Check sheet for the modelled part. Datum: model origin and axes. Units: mm. A direction names the side the tool comes from. Round coordinates to 2 decimals unless told otherwise and drop trailing zeros. Loops run counter-clockwise (first coordinate to the right, second up) from the corner with the lowest first, then second, coordinate; pieces in that order, holes last. Notation, with made-up numbers: (68.25, 72.5) -> (86.25, 72.5) arc R23 ccw to (86.25, 84.5) -> close; hole circle Ø5 at (42.25, -20). An arc over 180 degrees is marked (long way). Use one line per item in the form item = value. Start each with the question number.
(1) Draft check along Y on faces 1 (the flat face through (40.417, -66, 7)), 2 (the flat face through (42.917, -33, 8)), 3 (the flat face through (47, -54.781, 8)). Enter one of: released by +Y, released by -Y, zero draft, split by the parting line, or undercut.
(2) Go/stop test with flat-tipped pins: pin 1 (10 mm diameter, centred on x = 53.92, y = -49.38, fed in from +Z); pin 2 (4.5 mm diameter, centred on y = -59.5, z = 5.5, fed in from -X); pin 3 (5.5 mm diameter, centred on y = -29, z = 5, fed in from +X); pin 4 (3.5 mm diameter, centred on y = -35, z = 7, fed in from -X). Record where each tip stops, or that it passes through.
(3) Material ranges on probe 1 along X at (y, z) = (-62.5, 6); probe 2 along X at (y, z) = (-61, 10); probe 3 along X at (y, z) = (-59.5, 7.5), recorded low to high. Write a range as [from, to].
(4) Sectioned sample at C-C (y = -37). Record the cut outline in (x, z), and give its area (4 significant figures).
(5) Set-up check for faces 4 (the flat face through (48, -62.281, 5.7)), 5 (the flat face through (12, -23, 3.75)), 6 (the flat face through (39, -45.781, 7)), 7 (the flat face through (55, -45.781, 7)), 8 (the flat face through (12, -23, 11.25)): record each of +Z, -Z, +X, -X, +Y, -Y from which the full face is reachable in a straight line by a thin tool's end or side.
(6) Sectioned sample at B-B (x = 8). Record the cut outline in (y, z), and give its area (4 significant figures).
(7) Sectioned sample at A-A (z = 7.5). Record the cut outline in (x, y) (3 decimals), and give its area (3 significant figures).
from build123d import *

# Parameters (mm, degrees)
SKETCH1_R           = 3.175
PUSHER_BASE_DEPTH   = 15
SKETCH3_R           = 1.95
SCREW_HOLE_DEPTH    = 7.5
SKETCH6_W           = 7.5
SKETCH6_H           = 26.5
PUSHER_HEAD_DEPTH   = 3.75
FILLET1_R           = 6
FILLET5_R           = 6
FILLET6_R           = 6
SKETCH8_W           = 92.5
SKETCH8_H           = 4.5
BOSS_EXTRUDE1_DEPTH = 7.5


with BuildPart() as part:
    # Sketch1 → pusher base (new body)
    with BuildSketch(Plane.XY):
        Polygon((59.166899441, -45.781018283), (51.666899441, -45.781018283), (41.666899441, -45.781018283), (34.166899441, -45.781018283), (34.166899441, -69.281018283), (40.416899441, -69.281018283), (40.416899441, -62.281018283), (52.916899441, -62.281018283), (52.916899441, -69.281018283), (59.166899441, -69.281018283), align=None)
        with Locations((39.416899441, -49.381018283)):
            Circle(SKETCH1_R, mode=Mode.SUBTRACT)
        with Locations((53.916899441, -49.381018283)):
            Circle(SKETCH1_R, mode=Mode.SUBTRACT)
    extrude(amount=PUSHER_BASE_DEPTH)

    # Sketch3 → screw hole (cut)
    with BuildSketch(Plane.XZ.offset(62.281018283)):
        with Locations(Location((46.666899441, 7.5, 0), (0, 0, 270))):
            Circle(SKETCH3_R)
    extrude(amount=-SCREW_HOLE_DEPTH, mode=Mode.SUBTRACT)

    # Sketch6 → pusher head (add, symmetric)
    with BuildSketch(Plane.XY.offset(7.5)):
        with Locations((46.666899441, -32.531018283)):
            Rectangle(SKETCH6_W, SKETCH6_H)
    extrude(amount=PUSHER_HEAD_DEPTH, both=True)

    # Fillet1
    # the kernel refuses this fillet: 6 mm, written as the material it takes off along each edge
    with BuildSketch(Plane(origin=(74.166899441, -45.781018283, 0), x_dir=(0, 0, 1), z_dir=(-1, 0, 0))) as fillet1_piece_1_section:
        with BuildLine():
            CenterArc((FILLET1_R, -FILLET1_R), FILLET1_R, 90, 90)
            Line((0, -FILLET1_R), (0, 0))
            Line((0, 0), (FILLET1_R, 0))
        make_face()
    fillet1_piece_1 = extrude(amount=55, mode=Mode.PRIVATE)
    fillet1_piece_1 = split(fillet1_piece_1, bisect_by=Plane(origin=(62.291899441, -45.824840722, 3.75), z_dir=(0, 0, 1)), keep=Keep.TOP, mode=Mode.PRIVATE)
    fillet1_piece_1 = split(fillet1_piece_1, bisect_by=Plane(origin=(50.416899441, -45.824840722, 4.566140917), z_dir=(1, 0, 0)), keep=Keep.TOP, mode=Mode.PRIVATE)
    add(fillet1_piece_1, mode=Mode.SUBTRACT)
    with BuildSketch(Plane(origin=(74.166899441, -45.781018283, 0), x_dir=(0, 0, 1), z_dir=(-1, 0, 0))) as fillet1_piece_2_section:
        with BuildLine():
            CenterArc((FILLET1_R, -FILLET1_R), FILLET1_R, 90, 90)
            Line((0, -FILLET1_R), (0, 0))
            Line((0, 0), (FILLET1_R, 0))
        make_face()
    fillet1_piece_2 = extrude(amount=55, mode=Mode.PRIVATE)
    fillet1_piece_2 = split(fillet1_piece_2, bisect_by=Plane(origin=(62.291899441, -47.230240291, 3.75), z_dir=(0, 0, -1)), keep=Keep.TOP, mode=Mode.PRIVATE)
    fillet1_piece_2 = split(fillet1_piece_2, bisect_by=Plane(origin=(50.416899441, -47.230240291, 1.136674626), z_dir=(1, 0, 0)), keep=Keep.TOP, mode=Mode.PRIVATE)
    add(fillet1_piece_2, mode=Mode.SUBTRACT)
    with BuildSketch(Plane(origin=(74.166899441, -45.781018283, 0), x_dir=(0, 0, 1), z_dir=(-1, 0, 0))) as fillet1_piece_3_section:
        with BuildLine():
            CenterArc((FILLET1_R, -FILLET1_R), FILLET1_R, 90, 90)
            Line((0, -FILLET1_R), (0, 0))
            Line((0, 0), (FILLET1_R, 0))
        make_face()
    fillet1_piece_3 = extrude(amount=55, mode=Mode.PRIVATE)
    fillet1_piece_3 = split(fillet1_piece_3, bisect_by=Plane(origin=(46.666899441, -47.230240291, 3.75), z_dir=(0, 0, -1)), keep=Keep.TOP, mode=Mode.PRIVATE)
    fillet1_piece_3 = split(fillet1_piece_3, bisect_by=Plane(origin=(50.416899441, -47.230240291, 1.136674626), z_dir=(-1, 0, 0)), keep=Keep.TOP, mode=Mode.PRIVATE)
    fillet1_piece_3 = split(fillet1_piece_3, bisect_by=Plane(origin=(42.916899441, -47.230240291, 1.136674626), z_dir=(1, 0, 0)), keep=Keep.TOP, mode=Mode.PRIVATE)
    add(fillet1_piece_3, mode=Mode.SUBTRACT)
    with BuildSketch(Plane(origin=(74.166899441, -45.781018283, 0), x_dir=(0, 0, 1), z_dir=(-1, 0, 0))) as fillet1_piece_4_section:
        with BuildLine():
            CenterArc((FILLET1_R, -FILLET1_R), FILLET1_R, 90, 90)
            Line((0, -FILLET1_R), (0, 0))
            Line((0, 0), (FILLET1_R, 0))
        make_face()
    fillet1_piece_4 = extrude(amount=55, mode=Mode.PRIVATE)
    fillet1_piece_4 = split(fillet1_piece_4, bisect_by=Plane(origin=(31.041899441, -45.824840722, 3.75), z_dir=(0, 0, 1)), keep=Keep.TOP, mode=Mode.PRIVATE)
    fillet1_piece_4 = split(fillet1_piece_4, bisect_by=Plane(origin=(42.916899441, -45.824840722, 4.566140917), z_dir=(-1, 0, 0)), keep=Keep.TOP, mode=Mode.PRIVATE)
    add(fillet1_piece_4, mode=Mode.SUBTRACT)
    with BuildSketch(Plane(origin=(74.166899441, -45.781018283, 0), x_dir=(0, 0, 1), z_dir=(-1, 0, 0))) as fillet1_piece_5_section:
        with BuildLine():
            CenterArc((FILLET1_R, -FILLET1_R), FILLET1_R, 90, 90)
            Line((0, -FILLET1_R), (0, 0))
            Line((0, 0), (FILLET1_R, 0))
        make_face()
    fillet1_piece_5 = extrude(amount=55, mode=Mode.PRIVATE)
    fillet1_piece_5 = split(fillet1_piece_5, bisect_by=Plane(origin=(31.041899441, -47.230240291, 3.75), z_dir=(0, 0, -1)), keep=Keep.TOP, mode=Mode.PRIVATE)
    fillet1_piece_5 = split(fillet1_piece_5, bisect_by=Plane(origin=(42.916899441, -47.230240291, 1.136674626), z_dir=(-1, 0, 0)), keep=Keep.TOP, mode=Mode.PRIVATE)
    add(fillet1_piece_5, mode=Mode.SUBTRACT)
    with BuildSketch(Plane(origin=(19.166899441, -45.781018283, 15), x_dir=(0, 0, -1), z_dir=(1, 0, 0))) as fillet1_piece_6_section:
        with BuildLine():
            CenterArc((FILLET1_R, -FILLET1_R), FILLET1_R, 90, 90)
            Line((0, -FILLET1_R), (0, 0))
            Line((0, 0), (FILLET1_R, 0))
        make_face()
    fillet1_piece_6 = extrude(amount=55, mode=Mode.PRIVATE)
    fillet1_piece_6 = split(fillet1_piece_6, bisect_by=Plane(origin=(31.041899441, -45.824840722, 11.25), z_dir=(0, 0, -1)), keep=Keep.TOP, mode=Mode.PRIVATE)
    fillet1_piece_6 = split(fillet1_piece_6, bisect_by=Plane(origin=(42.916899441, -45.824840722, 10.433859083), z_dir=(-1, 0, 0)), keep=Keep.TOP, mode=Mode.PRIVATE)
    add(fillet1_piece_6, mode=Mode.SUBTRACT)
    with BuildSketch(Plane(origin=(19.166899441, -45.781018283, 15), x_dir=(0, 0, -1), z_dir=(1, 0, 0))) as fillet1_piece_7_section:
        with BuildLine():
            CenterArc((FILLET1_R, -FILLET1_R), FILLET1_R, 90, 90)
            Line((0, -FILLET1_R), (0, 0))
            Line((0, 0), (FILLET1_R, 0))
        make_face()
    fillet1_piece_7 = extrude(amount=55, mode=Mode.PRIVATE)
    fillet1_piece_7 = split(fillet1_piece_7, bisect_by=Plane(origin=(31.041899441, -47.230240291, 11.25), z_dir=(0, 0, 1)), keep=Keep.TOP, mode=Mode.PRIVATE)
    fillet1_piece_7 = split(fillet1_piece_7, bisect_by=Plane(origin=(42.916899441, -47.230240291, 13.863325374), z_dir=(-1, 0, 0)), keep=Keep.TOP, mode=Mode.PRIVATE)
    add(fillet1_piece_7, mode=Mode.SUBTRACT)
    with BuildSketch(Plane(origin=(19.166899441, -45.781018283, 15), x_dir=(0, 0, -1), z_dir=(1, 0, 0))) as fillet1_piece_8_section:
        with BuildLine():
            CenterArc((FILLET1_R, -FILLET1_R), FILLET1_R, 90, 90)
            Line((0, -FILLET1_R), (0, 0))
            Line((0, 0), (FILLET1_R, 0))
        make_face()
    fillet1_piece_8 = extrude(amount=55, mode=Mode.PRIVATE)
    fillet1_piece_8 = split(fillet1_piece_8, bisect_by=Plane(origin=(50.416899441, -47.230240291, 13.863325374), z_dir=(-1, 0, 0)), keep=Keep.TOP, mode=Mode.PRIVATE)
    fillet1_piece_8 = split(fillet1_piece_8, bisect_by=Plane(origin=(46.666899441, -47.230240291, 11.25), z_dir=(0, 0, 1)), keep=Keep.TOP, mode=Mode.PRIVATE)
    fillet1_piece_8 = split(fillet1_piece_8, bisect_by=Plane(origin=(42.916899441, -47.230240291, 13.863325374), z_dir=(1, 0, 0)), keep=Keep.TOP, mode=Mode.PRIVATE)
    add(fillet1_piece_8, mode=Mode.SUBTRACT)
    with BuildSketch(Plane(origin=(19.166899441, -45.781018283, 15), x_dir=(0, 0, -1), z_dir=(1, 0, 0))) as fillet1_piece_9_section:
        with BuildLine():
            CenterArc((FILLET1_R, -FILLET1_R), FILLET1_R, 90, 90)
            Line((0, -FILLET1_R), (0, 0))
            Line((0, 0), (FILLET1_R, 0))
        make_face()
    fillet1_piece_9 = extrude(amount=55, mode=Mode.PRIVATE)
    fillet1_piece_9 = split(fillet1_piece_9, bisect_by=Plane(origin=(50.416899441, -45.824840722, 10.433859083), z_dir=(1, 0, 0)), keep=Keep.TOP, mode=Mode.PRIVATE)
    fillet1_piece_9 = split(fillet1_piece_9, bisect_by=Plane(origin=(62.291899441, -45.824840722, 11.25), z_dir=(0, 0, -1)), keep=Keep.TOP, mode=Mode.PRIVATE)
    add(fillet1_piece_9, mode=Mode.SUBTRACT)
    with BuildSketch(Plane(origin=(19.166899441, -45.781018283, 15), x_dir=(0, 0, -1), z_dir=(1, 0, 0))) as fillet1_piece_10_section:
        with BuildLine():
            CenterArc((FILLET1_R, -FILLET1_R), FILLET1_R, 90, 90)
            Line((0, -FILLET1_R), (0, 0))
            Line((0, 0), (FILLET1_R, 0))
        make_face()
    fillet1_piece_10 = extrude(amount=55, mode=Mode.PRIVATE)
    fillet1_piece_10 = split(fillet1_piece_10, bisect_by=Plane(origin=(50.416899441, -47.230240291, 13.863325374), z_dir=(1, 0, 0)), keep=Keep.TOP, mode=Mode.PRIVATE)
    fillet1_piece_10 = split(fillet1_piece_10, bisect_by=Plane(origin=(62.291899441, -47.230240291, 11.25), z_dir=(0, 0, 1)), keep=Keep.TOP, mode=Mode.PRIVATE)
    add(fillet1_piece_10, mode=Mode.SUBTRACT)

    # Fillet5
    fillet5_edges = [part.edges().sort_by_distance(p)[0] for p in [
        (46.666899441, -46.218869418, 11.25),
    ]]
    fillet(fillet5_edges, radius=FILLET5_R)

    # Fillet6
    fillet6_edges = [part.edges().sort_by_distance(p)[0] for p in [
        (46.666899441, -46.218869418, 3.75),
    ]]
    fillet(fillet6_edges, radius=FILLET6_R)

    # Sketch8 → Boss-Extrude1 (add)
    with BuildSketch(Plane(origin=(0, 0, 3.75), x_dir=(-1, 0, 0), z_dir=(0, 0, -1))):
        with Locations((3.333100559, -21.531018283)):
            Rectangle(SKETCH8_W, SKETCH8_H)
    extrude(amount=-BOSS_EXTRUDE1_DEPTH)


solid = part.part
Checks:
q1.face_1 = zero draft
q1.face_2 = undercut
q1.face_3 = released by -Y
q2.pin_1 = 15
q2.pin_2 = 34.17
q2.pin_3 = 50.42
q2.pin_4 = 42.92
q3.probe_1 = [34.17, 40.42], [52.92, 59.17]
q3.probe_2 = [34.17, 59.17]
q3.probe_3 = [34.17, 44.72], [48.62, 59.17]
q4.outline = (42.92, 3.75) -> (50.42, 3.75) -> (50.42, 11.25) -> (42.92, 11.25) -> close
q4.area = 56.25 mm2
q5.face_4 = +Z, -Z, -Y
q5.face_5 = -Z, +X, -X, +Y
q5.face_6 = +Z, -Z, -X
q5.face_7 = +Z, -Z, +X, +Y
q5.face_8 = +Z, +X, -X, +Y
q6.outline = (-23.78, 3.75) -> (-19.28, 3.75) -> (-19.28, 11.25) -> (-23.78, 11.25) -> close
q6.area = 33.75 mm2
q7.outline = (-49.583, -23.781) -> (42.917, -23.781) -> (42.917, -45.781) -> (34.167, -45.781) -> (34.167, -69.281) -> (40.417, -69.281) -> (40.417, -62.281) -> (44.717, -62.281) -> (44.717, -54.781) -> (48.617, -54.781) -> (48.617, -62.281) -> (52.917, -62.281) -> (52.917, -69.281) -> (59.167, -69.281) -> (59.167, -45.781) -> (50.417, -45.781) -> (50.417, -19.281) -> (-49.583, -19.281) -> close; hole circle Ø6.35 at (39.417, -49.381); hole circle Ø6.35 at (53.917, -49.381)
q7.area = 1,020 mm2
